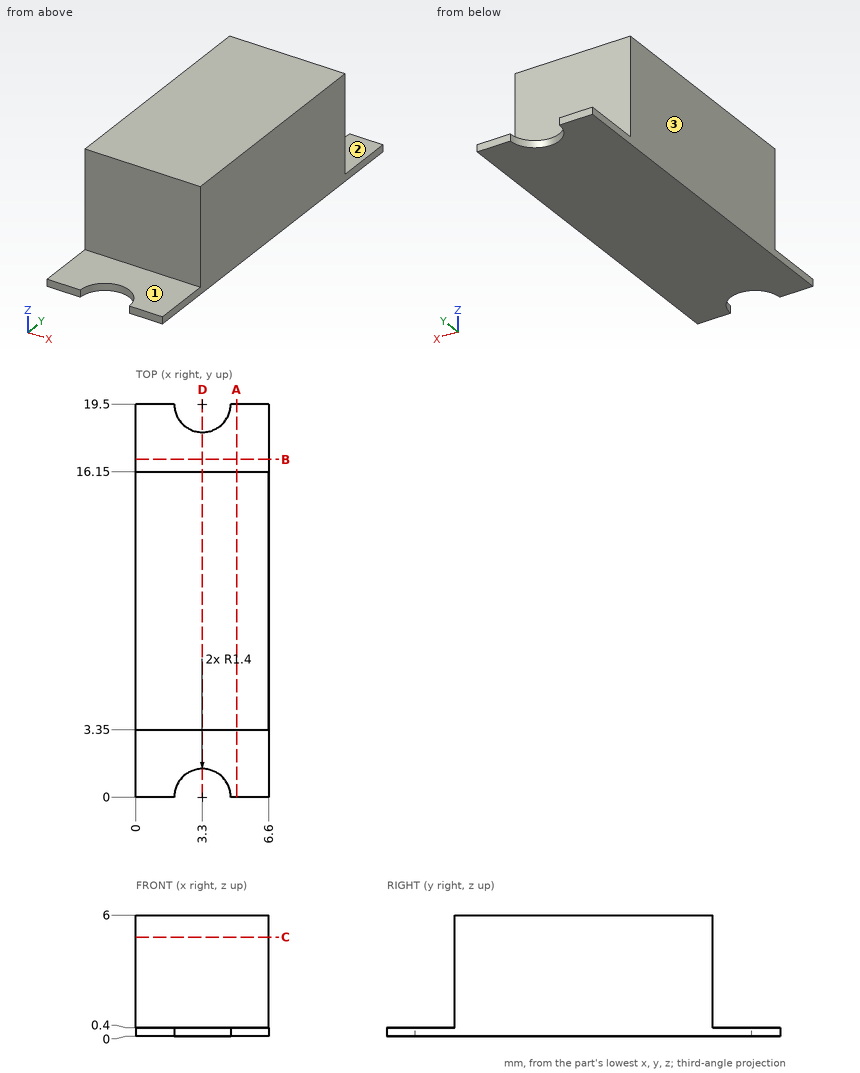
Design review of the part shown in the three views and the two pictorial views. Dimensions are in mm from the part's minimum x, y and z. A direction names the side the tool comes from. Round coordinates to 2 decimals unless told otherwise and drop trailing zeros. Loops run counter-clockwise (first coordinate to the right, second up) from the corner with the lowest first, then second, coordinate; pieces in that order, holes last. Notation, with made-up numbers: (-9, 58) -> (44, 58) arc R21 cw to (44, 94) -> close; hole circle Ø10 at (-8.5, -32). An arc over 180 degrees is marked (long way). Use one line per item in the form item = value. Start each with the question number.
Q1. Wall thickness on line 1 along Y through (x, z) = (2, 5.2); line 2 along Z through (x, y) = (4.75, 2.5): over which ranges is each line inside the solid? List them lowest first. Write a range as [from, to].
Q2. We need section D-D on x = 3.3. Give the boundary of the cut face in (y, z).
Q3. Machinability: for the marked faces 1, 2 and 3, which of the approach directions +Z, -Z, +X, -X, +Y, -Y give a long, thin tool a straight path to every point of the face, cutting with its end or side? Answer none if there is none.
Q4. We need section C-C on z = 4.9. Give the boundary of the cut face in (x, y), then the cut area to 3 significant figures.
Q5. We need section A-A on x = 5. Give the boundary of the cut face in (y, z), then the cut area to 3 significant figures.
Q6. For pin 1 Ø1.5 at (x, z) = (6, 4.5) entering from -Y; pin 2 Ø1.7 at (x, y) = (2, 1.5) entering from +Z; pin 3 Ø3 at (x, z) = (4.5, 2.5) entering from +Y, all flat-tipped, find the tip position at first contact; note any pin that passes through.
Q7. We need section B-B on y = 16.75. Give the boundary of the cut face in (x, z).
Calculated:
q1.line_1 = [3.35, 16.15]
q1.line_2 = [0, 0.4]
q2.outline = (1.4, 0) -> (18.1, 0) -> (18.1, 0.4) -> (16.15, 0.4) -> (16.15, 6) -> (3.35, 6) -> (3.35, 0.4) -> (1.4, 0.4) -> close
q3.face_1 = +Z, +X, -X, -Y
q3.face_2 = +Z, +X, -X, +Y
q3.face_3 = +Z, -Z, -X, +Y, -Y
q4.outline = (0, 3.35) -> (6.6, 3.35) -> (6.6, 16.15) -> (0, 16.15) -> close
q4.area = 84.5 mm²
q5.outline = (0, 0) -> (19.5, 0) -> (19.5, 0.4) -> (16.15, 0.4) -> (16.15, 6) -> (3.35, 6) -> (3.35, 0.4) -> (0, 0.4) -> close
q5.area = 79.5 mm²
q6.pin_1 = 3.35
q6.pin_2 = 0.4
q6.pin_3 = 16.15
q7.outline = (0, 0) -> (6.6, 0) -> (6.6, 0.4) -> (0, 0.4) -> close
